Study the drawing (mm; zero at the part's minimum x, y, z) and answer. A direction names the side the tool comes from. Coordinates: 2 decimals unless noted, no trailing zeros. Loops run counter-clockwise (first coordinate to the right, second up) from the corner with the lowest first, then second, coordinate; pieces in that order, holes last. Notation, with made-up numbers: (71, 19.5) - (102, 19.5) arc R25 ccw to (102, 56.5) - close; hole circle Ø2 at (-12.75, 28.25). An arc over 180 degrees is marked (long way). Use one line per item in the form item = value. Start each with the question number.
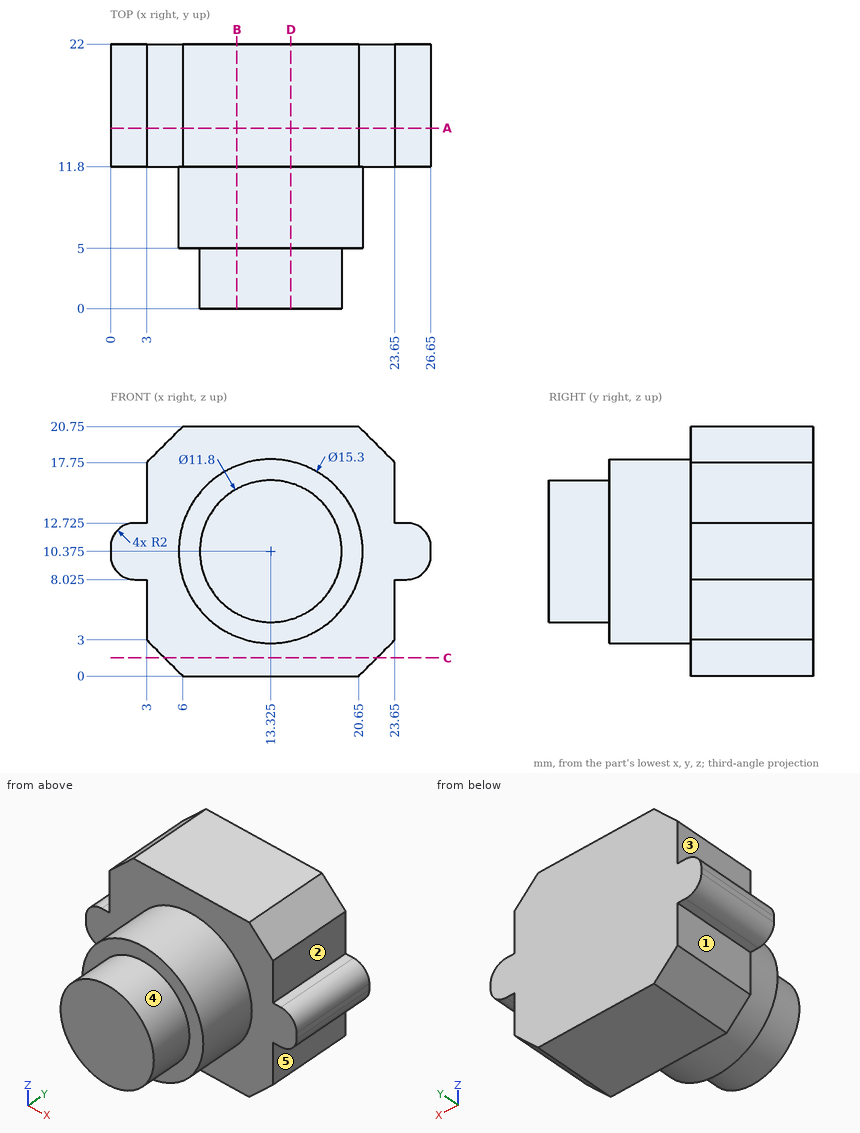
(1) A cutting plane is placed at C-C (z = 1.5). Determine the outline of the cut face in (x, y), then the cut area to 3 significant figures.
(2) Find the intervals of material crossed by probe 1 along Z at (x, y) = (24, 16.25) (3 decimals); probe 2 along X at (y, z) = (19.25, 5.75); probe 3 along Y at (x, z) = (6, 10.25), in increasing order. Write a range as from..to.
(3) For the marked faces 1, 2, 3, 4 and 5, determine the directions among +Z, -Z, +X, -X, +Y, -Y from which every point of the face is accessible in a straight line to the end or side of a thin tool.
(4) Each of these flat-tipped pins is pushed along its axis until it touches: pin 1 Ø4 at (y, z) = (18.5, 14.5) entering from +X; pin 2 Ø3 at (x, y) = (22.5, 4.5) entering from +Z; pin 3 Ø0.5 at (x, y) = (2.5, 18) entering from -Z (3 decimals); pin 4 Ø3 at (y, z) = (7.5, 5) entering from +X. Where does it stop, or does it pass through?
(5) A cutting plane is placed at A-A (y = 15). Determine the outline of the cut face in (x, z) (3 decimals).
(6) A cutting plane is placed at D-D (x = 15). Determine the outline of the cut face in (y, z), then the cut area to 3 significant figures.
(7) A cutting plane is placed at B-B (x = 10.5). Determine the outline of the cut face in (y, z).
Evaluation:
q1.outline = (4.5, 11.8) - (22.15, 11.8) - (22.15, 22) - (4.5, 22) - close
q1.area = 180 mm^2
q2.probe_1 = 8.025..12.725
q2.probe_2 = 3..23.65
q2.probe_3 = 5..22
q3.face_1 = -Z, -X, +Y, -Y
q3.face_2 = +Z, +X, +Y, -Y
q3.face_3 = +Z, -X, +Y, -Y
q3.face_4 = -Y
q3.face_5 = -Z, +X, +Y, -Y
q4.pin_1 = 25.57
q4.pin_2 = through
q4.pin_3 = 8.025
q4.pin_4 = 19.92
q5.outline = (0, 10.025) arc R2 ccw to (2, 8.025) - (3, 8.025) - (3, 3) - (6, 0) - (20.65, 0) - (23.65, 3) - (23.65, 8.025) - (24.65, 8.025) arc R2 ccw to (26.65, 10.025) - (26.65, 10.725) arc R2 ccw to (24.65, 12.725) - (23.65, 12.725) - (23.65, 17.75) - (20.65, 20.75) - (6, 20.75) - (3, 17.75) - (3, 12.725) - (2, 12.725) arc R2 ccw to (0, 10.725) - close
q6.outline = (0, 4.72) - (5, 4.72) - (5, 2.91) - (11.8, 2.91) - (11.8, 0) - (22, 0) - (22, 20.75) - (11.8, 20.75) - (11.8, 17.84) - (5, 17.84) - (5, 16.03) - (0, 16.03) - close
q6.area = 370 mm^2
q7.outline = (0, 5.2) - (5, 5.2) - (5, 3.27) - (11.8, 3.27) - (11.8, 0) - (22, 0) - (22, 20.75) - (11.8, 20.75) - (11.8, 17.48) - (5, 17.48) - (5, 15.55) - (0, 15.55) - close
